```python
from build123d import *

# Parameters (mm, degrees)
F0_W     = 139.704422
F0_H     = 82.653814
F0_W_2   = 130.242362
F0_H_2   = 72.07857
F1_DEPTH = 43.434
F2_R     = 9.957557
F3_DEPTH = 170.434
F4_W     = 65.121188
F4_H     = 53.194226
F5_DEPTH = 111.252


with BuildPart() as f1:
    # F0 (on Top) → F1 (new body, symmetric)
    with BuildSketch(Plane.XY):
        Rectangle(F0_W, F0_H)
        Rectangle(F0_W_2, F0_H_2, mode=Mode.SUBTRACT)
    extrude(amount=F1_DEPTH, both=True)

    # F2 (on face) → F3 (cut)
    with BuildSketch(Plane.YZ.offset(69.852211)):
        Circle(F2_R)
    extrude(amount=-F3_DEPTH, mode=Mode.SUBTRACT)

    # F4 (on face) → F5 (cut)
    with BuildSketch(Plane.XZ.offset(41.326907)):
        with Locations((0, 43.434)):
            Rectangle(F4_W, F4_H)
    extrude(amount=-F5_DEPTH, mode=Mode.SUBTRACT)


solid = f1.part
```
The model under review builds one solid part; all positions refer to its coordinate system, in mm. A direction names the side the tool comes from. Round coordinates to 2 decimals unless told otherwise and drop trailing zeros. Loops run counter-clockwise (first coordinate to the right, second up) from the corner with the lowest first, then second, coordinate; pieces in that order, holes last. Notation, with made-up numbers: M 72,76.5 L 125,76.5 A18 cw 125,87.5 Z; hole C 66.25,-19 d1. An arc over 180 degrees is marked long. Answer as a JSON object with one key per item and string values.
(1) Clearance check with flat-ended pins moving along their axes: P1, Ø4, axis at x = 12.5, y = 39.5, coming from the +Z side; P2, Ø12, axis at y = 0, z = 0, coming from the -X side; P3, Ø8, axis at x = 39.5, y = 32.5, coming from the +Z side. State where each tip first meets the part, or that it passes through.
Resolved:
{"P1": "z = 16.84", "P2": "through", "P3": "z = 43.43"}
(2) Take a section at D-D on y = -16. Give the boundary of the cut face in (x, z).
Resolved:
{"outline": "M -69.85,-43.43 L -65.12,-43.43 L -65.12,43.43 L -69.85,43.43 Z; M 65.12,-43.43 L 69.85,-43.43 L 69.85,43.43 L 65.12,43.43 Z"}
(3) Tool access review of faces 4 (the flat face through (-65.121, -0.5, 10.3)), 5 (the flat face through (0, 39, 16.837)), 6 (the cylindrical face through (67.52, 5.35, 8.4)): name each direction out of +Z, -Z, +X, -X, +Y, -Y from which nothing blocks a thin tool from reaching the whole face with its end or side.
Resolved:
{"face 4": "+Z, -Z", "face 5": "+Z, +Y, -Y", "face 6": "+X, -X"}
(4) Take a section at B-B on z = 0. Give the boundary of the cut face in (x, y), and give its area (3 significant figures).
Resolved:
{"outline": "M -69.85,-41.33 L 69.85,-41.33 L 69.85,-9.96 L 65.12,-9.96 L 65.12,-36.04 L -65.12,-36.04 L -65.12,-9.96 L -69.85,-9.96 Z; M -69.85,9.96 L -65.12,9.96 L -65.12,36.04 L 65.12,36.04 L 65.12,9.96 L 69.85,9.96 L 69.85,41.33 L -69.85,41.33 Z", "area": "1,970 mm²"}
(5) To check wall thickness, follow line 1 along Y through (x, z) = (16.5, -5.5); line 2 along X through (y, z) = (-7, -39); line 3 along Z through (x, y) = (-68.25, 0). State the ranges of each line that lie inside material, in increasing order.
Resolved:
{"line 1": "-41.33 to -36.04, 36.04 to 41.33", "line 2": "-69.85 to -65.12, 65.12 to 69.85", "line 3": "-43.43 to -9.96, 9.96 to 43.43"}
(6) Take a section at C-C on x = -30. Give the boundary of the cut face in (y, z), and give its area (3 significant figures).
Resolved:
{"outline": "M -41.33,-43.43 L -36.04,-43.43 L -36.04,16.84 L -41.33,16.84 Z; M 36.04,-43.43 L 41.33,-43.43 L 41.33,16.84 L 36.04,16.84 Z", "area": "637 mm²"}
(7) Take a section at A-A on y = 0. Give the boundary of the cut face in (x, z).
Resolved:
{"outline": "M -69.85,-43.43 L -65.12,-43.43 L -65.12,-9.96 L -69.85,-9.96 Z; M -69.85,9.96 L -65.12,9.96 L -65.12,43.43 L -69.85,43.43 Z; M 65.12,-43.43 L 69.85,-43.43 L 69.85,-9.96 L 65.12,-9.96 Z; M 65.12,9.96 L 69.85,9.96 L 69.85,43.43 L 65.12,43.43 Z"}
(8) Draft analysis for pull direction X (two halves, no side actions). For faces 1 (the flat face through (-69.852, -0.6, 10.3)), 2 (the flat face through (32.561, 39, 30)), 3 (the flat face through (-6, -37, -43.434)), state which applies: released by +X, released by -X, zero draft, split by the parting line, or undercut.
Resolved:
{"face 1": "released by -X", "face 2": "undercut", "face 3": "zero draft"}
